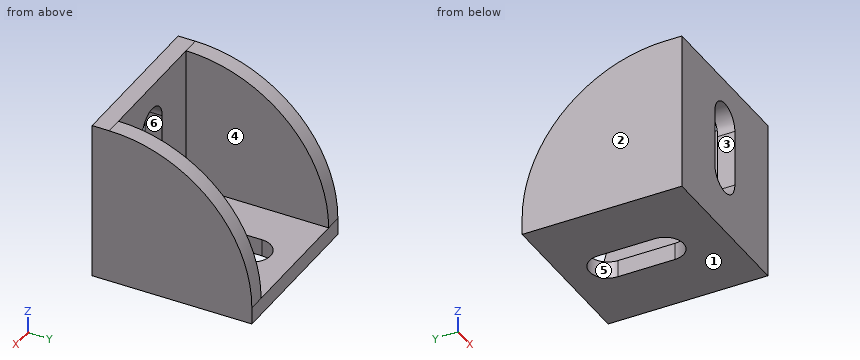
from build123d import *

# Parameters (mm, degrees)
SKETCH1_W           = 28
SKETCH1_H           = 28
BOSS_EXTRUDE1_DEPTH = 3
SKETCH2_W           = 28
SKETCH2_H           = 25
BOSS_EXTRUDE2_DEPTH = 3
BOSS_EXTRUDE3_DEPTH = 3
BOSS_EXTRUDE4_START = -3
BOSS_EXTRUDE4_DEPTH = 3
CUT_EXTRUDE1_DEPTH  = 3
CUT_EXTRUDE2_DEPTH  = 3


with BuildPart() as part:
    # Sketch1 → Boss-Extrude1 (new body)
    with BuildSketch(Plane(origin=(0, 0, 0), x_dir=(1, 0, 0), z_dir=(0, 1, 0))):
        with Locations((14, -14)):
            Rectangle(SKETCH1_W, SKETCH1_H)
    extrude(amount=BOSS_EXTRUDE1_DEPTH)

    # Sketch2 → Boss-Extrude2 (add)
    with BuildSketch(Plane(origin=(0, 0, 0), x_dir=(-1, 0, 0), z_dir=(0, 0, -1))):
        with Locations((-14, 15.5)):
            Rectangle(SKETCH2_W, SKETCH2_H)
    extrude(amount=-BOSS_EXTRUDE2_DEPTH)

    # Sketch3 → Boss-Extrude3 (add)
    with BuildSketch(Plane.ZY):
        with BuildLine():
            Line((3, 28), (3, 3))
            Line((3, 3), (28, 3))
            ThreePointArc((28, 3), (20.67766953, 20.67766953), (3, 28))
        make_face()
    extrude(amount=-BOSS_EXTRUDE3_DEPTH)

    # Sketch4 → Boss-Extrude4 (add)
    with BuildSketch(Plane(origin=(28, 0, 0), x_dir=(0, 0, -1), z_dir=(1, 0, 0)).offset(BOSS_EXTRUDE4_START)):
        with BuildLine():
            Line((-28, 3), (-3, 3))
            Line((-3, 3), (-3, 28))
            ThreePointArc((-3, 28), (-20.67766953, 20.67766953), (-28, 3))
        make_face()
    extrude(amount=BOSS_EXTRUDE4_DEPTH)

    # Sketch5 → Cut-Extrude1 (cut)
    with BuildSketch(Plane.XY.offset(3)):
        with BuildLine():
            Line((10.75, 10.5), (10.75, 20.5))
            ThreePointArc((10.75, 20.5), (14, 23.75), (17.25, 20.5))
            Line((17.25, 20.5), (17.25, 10.5))
            ThreePointArc((17.25, 10.5), (14, 7.25), (10.75, 10.5))
        make_face()
    extrude(amount=-CUT_EXTRUDE1_DEPTH, mode=Mode.SUBTRACT)

    # Sketch6 → Cut-Extrude2 (cut)
    with BuildSketch(Plane(origin=(0, 3, 0), x_dir=(1, 0, 0), z_dir=(0, 1, 0))):
        with BuildLine():
            Line((17.25, -10.5), (17.25, -20.5))
            ThreePointArc((17.25, -20.5), (14, -23.75), (10.75, -20.5))
            Line((10.75, -20.5), (10.75, -10.5))
            ThreePointArc((10.75, -10.5), (14, -7.25), (17.25, -10.5))
        make_face()
    extrude(amount=-CUT_EXTRUDE2_DEPTH, mode=Mode.SUBTRACT)


solid = part.part
Part model, mm, in its own coordinate system. Face numbers are marked on the shaded views. A direction names the side the tool comes from. Coordinates: 2 decimals unless noted, no trailing zeros. Order: outer loops, then holes, each group sorted by start corner. A loop starts at its lowest first (then second) coordinate and runs counter-clockwise, first axis right, second up.
(1) Tool access for the marked faces 4, 5 and 6: list every direction of +Z, -Z, +X, -X, +Y, -Y with a clear straight run to the whole face (end or side of a thin tool).
Check sheet entries:
face 4: +Z, +Y
face 5: +Z, -Z
face 6: +Y, -Y
(2) Slice it at A-A, the plane x = 12.75. Write the cut outline in (y, z).
Check sheet entries:
outline: (0, 0) - (7.5, 0) - (7.5, 3) - (3, 3) - (3, 7.5) - (0, 7.5) - close; (0, 23.5) - (3, 23.5) - (3, 28) - (0, 28) - close; (23.5, 0) - (28, 0) - (28, 3) - (23.5, 3) - close
(3) Probe L1, parallel to X at y = 13, z = 6.75; L2, parallel to X at y = 2.75, z = 19.75; L3, parallel to Z at x = 5, y = 10.75. List the from-to ranges inside material, lowest first.
Check sheet entries:
L1: x = 0 to 3, 25 to 28
L2: x = 0 to 10.75, 17.25 to 28
L3: z = 0 to 3
(4) Pull direction Z, two halves, no side cores. Call the marked faces 1, 2 and 3: pulls with the +Z half, pulls with the -Z half, needs draft (parallel to the pull), parting line crosses it, or undercut.
Check sheet entries:
face 1: pulls with the -Z half
face 2: needs draft
face 3: undercut
(5) Slice it at B-B, the plane y = 11. Write the cut outline in (x, z).
Check sheet entries:
outline: (0, 0) - (10.75, 0) - (10.75, 3) - (3, 3) - (3, 26.69) - (0, 26.69) - close; (17.25, 0) - (28, 0) - (28, 26.69) - (25, 26.69) - (25, 3) - (17.25, 3) - close
(6) Slice it at D-D, the plane x = 21.25. Write the cut outline in (y, z).
Check sheet entries:
outline: (0, 0) - (28, 0) - (28, 3) - (3, 3) - (3, 28) - (0, 28) - close
(7) Pin check, flat tips, straight feed: pin 1 Ø7.5 at (y, z) = (18.5, 13.5) entering from -X; pin 2 Ø6.5 at (x, z) = (11, 18.5) entering from +Y; pin 3 Ø6.5 at (x, y) = (16, 12) entering from +Z. Stop position of each tip, or through.
Check sheet entries:
pin 1: stops at x = 0
pin 2: stops at y = 3
pin 3: stops at z = 3
(8) Slice it at C-C, the plane z = 22.25. Write the cut outline in (x, y), and give its area (3 significant figures).
Check sheet entries:
outline: (0, 0) - (11.26, 0) - (11.26, 3) - (3, 3) - (3, 18.95) - (0, 18.95) - close; (16.74, 0) - (28, 0) - (28, 18.95) - (25, 18.95) - (25, 3) - (16.74, 3) - close
area: 163 mm2
